For this review, take the finished solid that the model builds, in its own axes (mm). A direction names the side the tool comes from. Give positions to 0.01 mm unless a question says otherwise; leave off trailing zeros. Write each loop counter-clockwise with the first axis right and the second up, starting at its lowest first coordinate (ties: lowest second). Pieces come first, ordered by that corner, then holes.
Q1. We need section D-D (y = 27). Write out the cut boundary in (x, z).
Q2. We need section A-A (y = 12.5). Write out the cut boundary in (x, z), then the cut area to 3 significant figures.
Q3. Machinability: for faces 1 (the flat face through (10, -25, -6)), 2 (the flat face through (12.5, 0, -11)), 3 (the flat face through (10, 25, -6)), 4 (the flat face through (-35, 0, 2)), which of the approach directions +Z, -Z, +X, -X, +Y, -Y give a long, thin tool a straight path to every point of the face, cutting with its end or side? Answer none if there is none.
Q4. We need section C-C (z = -1.5). Write out the cut boundary in (x, y), then the cut area to 3 significant figures.
Q5. Mouldability with a two-part tool opening along Y and no side actions: class faces 5 (the flat face through (0, 1, 0)), 6 (the cylindrical face through (-10.67, -25.9, -0.86)), 7 (the cylindrical face through (10.04, -13.65, -12.77)) as released by +Y, released by -Y, zero draft, split by the parting line, or undercut.
Q6. Insertion check: P1, Ø4, axis at x = -10.5, z = -5.5, coming from the -Y side; P2, Ø5, axis at x = 18.5, y = 14.5, coming from the -Z side; P3, Ø8, axis at y = 11, z = -17, coming from the +X side; P4, Ø10, axis at x = 16, y = 13, coming from the -Z side. Each pin has a flat end and moves straight along its axis. Give the tip position at first contact, or say it passes through.
Q7. For line 1 (Y direction, x = 8.95, z = -10); line 2 (X direction, y = 20.5, z = -3.75); line 3 (Z direction, x = 11, y = -12), list the stretches that pass through material, from the lowest coordinate up.
Q8. We need section B-B (x = 8.5). Write out the cut boundary in (y, z), then the cut area to 3 significant figures.
```python
from build123d import *

# Parameters (mm, degrees)
SKETCH1_W           = 70
SKETCH1_H           = 90
BOSS_EXTRUDE1_DEPTH = 5
SKETCH3_W           = 5
SKETCH3_H           = 50
BOSS_EXTRUDE2_DEPTH = 20
SKETCH4_R           = 3
CUT_EXTRUDE1_DEPTH  = 48.5
FILLET1_R           = 3
FILLET2_R           = 10
FILLET3_R           = 10


with BuildPart() as part:
    # Sketch1 → Boss-Extrude1 (new body)
    with BuildSketch(Plane.XY):
        Rectangle(SKETCH1_W, SKETCH1_H)
    extrude(amount=BOSS_EXTRUDE1_DEPTH)

    # Sketch3 → Boss-Extrude2 (add)
    with BuildSketch(Plane(origin=(0, 0, 0), x_dir=(-1, 0, 0), z_dir=(0, 0, -1))):
        with Locations((10, 0)):
            Rectangle(SKETCH3_W, SKETCH3_H)
        with Locations((-10, 0)):
            Rectangle(SKETCH3_W, SKETCH3_H)
    extrude(amount=BOSS_EXTRUDE2_DEPTH)

    # Sketch4 → Cut-Extrude1 (cut, through all)
    with BuildSketch(Plane(origin=(12.5, 0, 0), x_dir=(0, 0, -1), z_dir=(1, 0, 0))):
        with Locations((10, 12.5)):
            Circle(SKETCH4_R)
        with Locations((10, -12.5)):
            Circle(SKETCH4_R)
    extrude(amount=-CUT_EXTRUDE1_DEPTH, mode=Mode.SUBTRACT)

    # Fillet1
    fillet1_edges = [part.edges().sort_by_distance(p)[0] for p in [
        (10, 25, 0),
        (12.5, 0, 0),
        (10, -25, 0),
        (-12.5, 0, 0),
        (-10, 25, 0),
        (-10, -25, 0),
    ]]
    fillet(fillet1_edges, radius=FILLET1_R)

    # Fillet2
    fillet2_edges = [part.edges().sort_by_distance(p)[0] for p in [
        (10, 25, -20),
        (10, -25, -20),
        (-10, 25, -20),
        (-10, -25, -20),
    ]]
    fillet(fillet2_edges, radius=FILLET2_R)

    # Fillet3
    fillet3_edges = [part.edges().sort_by_distance(p)[0] for p in [
        (35, -45, 2.5),
        (-35, -45, 2.5),
        (-35, 45, 2.5),
        (35, 45, 2.5),
    ]]
    fillet(fillet3_edges, radius=FILLET3_R)


solid = part.part
```
Computed:
1. outline: (-35, 0) - (-15.5, 0) arc R3 cw to (-14.5, -0.17) - (-7.5, -0.17) - (-7.5, 0) - (7.5, 0) - (7.5, -0.17) - (14.5, -0.17) arc R3 cw to (15.5, 0) - (35, 0) - (35, 5) - (-35, 5) - close
2. outline: (-35, 0) - (-15.5, 0) arc R3 cw to (-12.5, -3) - (-12.5, -7) - (-7.5, -7) - (-7.5, 0) - (7.5, 0) - (7.5, -7) - (12.5, -7) - (12.5, -3) arc R3 cw to (15.5, 0) - (35, 0) - (35, 5) - (-35, 5) - close; (-12.5, -20) - (-7.5, -20) - (-7.5, -13) - (-12.5, -13) - close; (7.5, -20) - (12.5, -20) - (12.5, -13) - (7.5, -13) - close
2. area: 494 mm2
3. face 1: -Z, +X, -X, -Y
3. face 2: -Z, +X, +Y, -Y
3. face 3: -Z, +X, -X, +Y
3. face 4: +Z, -Z, -X, +Y, -Y
4. outline: (-12.9, -25.4) - (-7.5, -25.4) - (-7.5, 25.4) - (-12.9, 25.4) - close; (7.5, -25.4) - (12.9, -25.4) - (12.9, 25.4) - (7.5, 25.4) - close
4. area: 549 mm2
5. face 5: zero draft
5. face 6: released by -Y
5. face 7: undercut
6. P1: stops at y = -25
6. P2: stops at z = 0
6. P3: stops at x = 12.5
6. P4: stops at z = -20
7. line 1: y = -25 to -15.5, -9.5 to 9.5, 15.5 to 25
7. line 2: x = -12.5 to -7.5, 7.5 to 12.5
7. line 3: z = -20 to -12.96, -7.04 to 5
8. outline: (-45, 0) - (-28, 0) arc R3 cw to (-25, -3) - (-25, -10) arc R10 ccw to (-15, -20) - (15, -20) arc R10 ccw to (25, -10) - (25, -3) arc R3 cw to (28, 0) - (45, 0) - (45, 5) - (-45, 5) - close; hole circle Ø6 at (-12.5, -10); hole circle Ø6 at (12.5, -10)
8. area: 1,350 mm2
